The model under review builds one solid part; all positions refer to its coordinate system, in mm. Face numbers are marked on the shaded views. A direction names the side the tool comes from. Round coordinates to 2 decimals unless told otherwise and drop trailing zeros. Order: outer loops, then holes, each group sorted by start corner. A loop starts at its lowest first (then second) coordinate and runs counter-clockwise, first axis right, second up.
1) Machinability: for the marked faces 1 and 2, which of the approach directions +Z, -Z, +X, -X, +Y, -Y give a long, thin tool a straight path to every point of the face, cutting with its end or side? Answer none if there is none.
2) Mouldability with a two-part tool opening along X and no side actions: class the marked faces 3, 4 and 5 as pulls with the +X half, pulls with the -X half, needs draft (parallel to the pull), parting line crosses it, or undercut.
3) Consider section C-C (z = -5.75). Give the boundary of the cut face in (x, y).
4) Clearance check with flat-ended pins moving along their axes: P1, Ø5, axis at y = -3.5, z = -6, coming from the -X side; P2, Ø5, axis at y = -1.5, z = -9, coming from the +X side; P3, Ø3, axis at y = 2, z = -9, coming from the -X side. State where each tip first meets the part, or that it passes through.
5) To check wall thickness, follow L1, parallel to Y at x = 0, z = 1.35; L2, parallel to Y at x = 0, z = 1.15; L3, parallel to Z at x = -1.75, y = 4.5. State the ranges of each line that lie inside material, in increasing order.
6) Consider section A-A (y = 0). Give the boundary of the cut face in (x, z), then the cut area to 3 significant figures.
from build123d import *

# Parameters (mm, degrees)
F0_R     = 7
F0_R_2   = 6
F0_R_3   = 4.5
F1_DEPTH = 2
F2_SIZE  = 1.5
F3_DEPTH = 0.5
F4_R     = 4.25
F5_DEPTH = 3
F6_DEPTH = 12


with BuildPart() as f1:
    # F0 (on Top) → F1 (new body)
    with BuildSketch(Plane.XY):
        Circle(F0_R)
        Circle(F0_R_2, mode=Mode.SUBTRACT)
        Circle(F0_R_2)
        Circle(F0_R_3, mode=Mode.SUBTRACT)
    extrude(amount=F1_DEPTH)

    # F2
    f2_edges = [f1.edges().sort_by_distance(p)[0] for p in [
        (-7, 0, 2),
    ]]
    chamfer(f2_edges, length=F2_SIZE)

    # F0 (on Top) → F3 (join)
    with BuildSketch(Plane.XY):
        Circle(F0_R_3)
    extrude(amount=F3_DEPTH)

    # F4 (on face) → F5 (join)
    with BuildSketch(Plane.XY.offset(0.5)):
        Circle(F4_R)
    extrude(amount=F5_DEPTH)

    # F0 (on Top) → F6 (join)
    with BuildSketch(Plane.XY):
        Circle(F0_R_2)
        Circle(F0_R_3, mode=Mode.SUBTRACT)
        Circle(F0_R_3)
    extrude(amount=-F6_DEPTH)


solid = f1.part
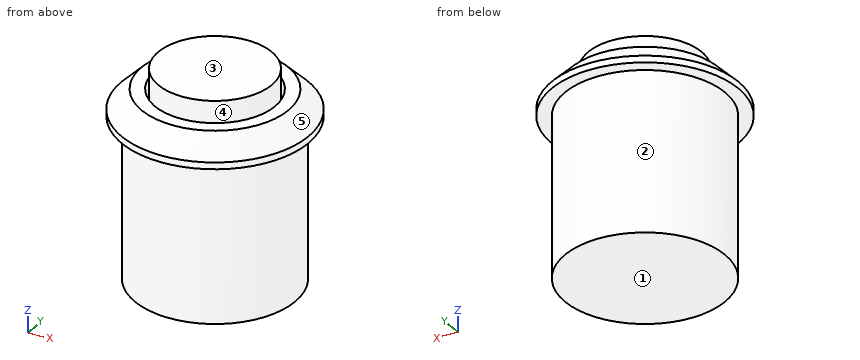
Answer below:
1. face 1: -Z, +X, -X, +Y, -Y
1. face 2: -Z
2. face 3: needs draft
2. face 4: undercut
2. face 5: parting line crosses it
3. outline: circle Ø12 at (0, 0)
4. P1: stops at x = -5.92
4. P2: stops at x = 6
4. P3: stops at x = -5.98
5. L1: y = -6.15 to -4.5, -4.25 to 4.25, 4.5 to 6.15
5. L2: y = -6.35 to -4.5, -4.25 to 4.25, 4.5 to 6.35
5. L3: z = -12 to 2
6. outline: (-7, 0) - (-6, 0) - (-6, -12) - (6, -12) - (6, 0) - (7, 0) - (7, 0.5) - (5.5, 2) - (4.5, 2) - (4.5, 0.5) - (4.25, 0.5) - (4.25, 3.5) - (-4.25, 3.5) - (-4.25, 0.5) - (-4.5, 0.5) - (-4.5, 2) - (-5.5, 2) - (-7, 0.5) - close
6. area: 182 mm2
